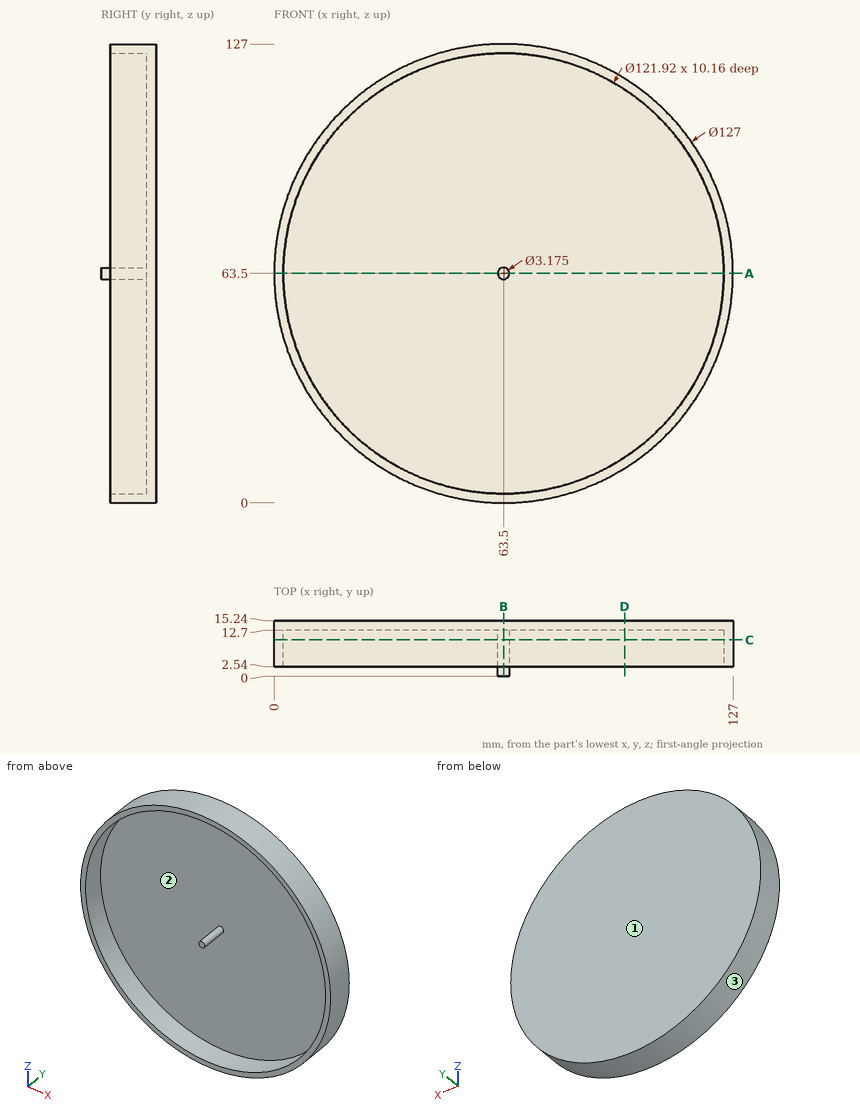
Could you check a few things on this drawing? It's one solid part, dimensions in mm from its lowest x, y, z. Round coordinates to 2 decimals unless told otherwise and drop trailing zeros. Order: outer loops, then holes, each group sorted by start corner. A loop starts at its lowest first (then second) coordinate and runs counter-clockwise, first axis right, second up.
Q1. Thinking about a two-plate mould opening in X: for the marked faces 1, 2 and 3, which applies, released by +X, released by -X, zero draft, split by the parting line, or undercut?
Geometry says:
face 1: zero draft
face 2: undercut
face 3: split by the parting line
Q2. Imagine slicing it at C-C, the plane y = 10. List the corners of the cut face in (x, z) for me (1 decimal), then the cut area to 3 significant figures.
Geometry says:
outline: circle Ø127 at (63.5, 63.5); circle Ø3.2 at (63.5, 63.5); hole circle Ø121.9 at (63.5, 63.5)
area: 1,000 mm2
Q3. Imagine slicing it at D-D, the plane x = 97. List the corners of the cut face in (y, z) for me, then the cut area to 3 significant figures.
Geometry says:
outline: (2.54, 9.56) - (15.24, 9.56) - (15.24, 117.44) - (2.54, 117.44) - (2.54, 114.43) - (12.7, 114.43) - (12.7, 12.57) - (2.54, 12.57) - close
area: 335 mm2
Q4. Imagine slicing it at B-B, the plane x = 63.5. List the corners of the cut face in (y, z) for me.
Geometry says:
outline: (0, 61.91) - (12.7, 61.91) - (12.7, 2.54) - (2.54, 2.54) - (2.54, 0) - (15.24, 0) - (15.24, 127) - (2.54, 127) - (2.54, 124.46) - (12.7, 124.46) - (12.7, 65.09) - (0, 65.09) - close
Q5. Imagine slicing it at A-A, the plane z = 63.5. List the corners of the cut face in (x, y) for me.
Geometry says:
outline: (0, 2.54) - (2.54, 2.54) - (2.54, 12.7) - (61.91, 12.7) - (61.91, 0) - (65.09, 0) - (65.09, 12.7) - (124.46, 12.7) - (124.46, 2.54) - (127, 2.54) - (127, 15.24) - (0, 15.24) - close
Q6. I'm going to push flat-ended pins straight in: P1, Ø12, axis at x = 111.5, z = 28, coming from the -Y side; P2, Ø1, axis at y = 3, z = 100.5, coming from the -X side; P3, Ø4, axis at x = 56.5, z = 61, coming from the -Y side. Where does each tip first touch, or does it pass through?
Geometry says:
P1: stops at y = 2.54
P2: stops at x = 11.54
P3: stops at y = 12.7
Q7. Please list where these lines run through material, in increasing order: probe 1 along Z at (x, y) = (63.5, 7.25); probe 2 along Y at (x, z) = (80, 34.5); probe 3 along X at (y, z) = (12, 101).
Geometry says:
probe 1: z = 0 to 2.54, 61.91 to 65.09, 124.46 to 127
probe 2: y = 12.7 to 15.24
probe 3: x = 12.26 to 15.44, 111.56 to 114.74
